Check sheet for the modelled part. Datum: model origin and axes. Units: mm. Face numbers are marked on the shaded views. A direction names the side the tool comes from. Round coordinates to 2 decimals unless told otherwise and drop trailing zeros. Write each loop counter-clockwise with the first axis right and the second up, starting at its lowest first coordinate (ties: lowest second). Pieces come first, ordered by that corner, then holes. Notation, with made-up numbers: (81.25, 35.25) - (131.25, 35.25) arc R24 ccw to (131.25, 61.25) - close; hole circle Ø9 at (-30.75, -13). An arc over 180 degrees is marked (long way). Answer as a JSON object with one key per item and string values. Group by question number.
Item 1: Sectioned sample at A-A on y = 0. Record the boundary of the cut face in (x, z), plus the area to 3 significant figures.
Item 2: Sectioned sample at D-D on y = -5.5. Record the boundary of the cut face in (x, z).
Item 3: Sectioned sample at C-C on x = 0. Record the boundary of the cut face in (y, z), plus the area to 3 significant figures.
Item 4: Sectioned sample at B-B on z = -35. Record the boundary of the cut face in (x, y), plus the area to 3 significant figures.
Item 5: Thickness scan on line 1 (Z direction, x = 4.5, y = -4.5); line 2 (X direction, y = 2.5, z = -33); line 3 (Y direction, x = 13.8, z = -35). Record the ranges inside material, lowest first.
Item 6: Gauge pin test, flat ends, axial feed: P1, Ø3.5, axis at x = 35.5, y = 2.5, coming from the +Z side; P2, Ø8, axis at y = 0, z = -35, coming from the +X side; P3, Ø6, axis at x = -35, z = 0, coming from the -Y side; P4, Ø1.5, axis at y = 5.5, z = 23, coming from the -X side. Record the tip position at first contact, or that the pin passes through.
Item 7: Release check for a two-part mould opening along X. For the marked faces 5, 6, 7 and 8 record: pulls with the +X half, pulls with the -X half, needs draft (parallel to the pull), parting line crosses it, or undercut.
Item 8: Set-up check for the marked faces 1, 2, 3 and 4: record each of +Z, -Z, +X, -X, +Y, -Y from which the full face is reachable in a straight line by a thin tool's end or side.
```python
from build123d import *

# Parameters (mm, degrees)
SCHIZZO1_R                    = 12
SCHIZZO1_R_2                  = 5
ESTRUSIONE_ESTRUSIONE1_DEPTH  = 7.5
TAGLIO_ESTRUSIONE1_DEPTH      = 73.284161474
TAGLIO_ESTRUSIONE1_DEPTH_BACK = 5
SCHIZZO3_R                    = 5
SCHIZZO4_R                    = 5
TAGLIO_ESTRUSIONE2_DEPTH      = 10
FORO_7_0_7_1_D                = 7
FORO_6_0_6_1_D                = 6


with BuildPart() as part:
    # Schizzo1 → Estrusione-Estrusione1 (new, symmetric)
    with BuildSketch(Plane(origin=(0, 0, 0), x_dir=(1, 0, 0), z_dir=(0, 1, 0))):
        with BuildLine():
            Line((-40, 30), (-16, 30))
            Line((-16, 30), (-16, 40))
            Line((-16, 40), (-10, 40))
            Line((-10, 40), (-10, 30))
            Line((-10, 30), (10, 30))
            Line((10, 30), (10, 40))
            Line((10, 40), (16, 40))
            Line((16, 40), (16, 30))
            Line((16, 30), (40, 30))
            ThreePointArc((40, 30), (0, -50), (-40, 30))
        make_face()
        with Locations(Location((0, 0, 0), (0, 0, 270))):
            Circle(SCHIZZO1_R, mode=Mode.SUBTRACT)
        with Locations(Location((0, -30, 0), (0, 0, 270))):
            Circle(SCHIZZO1_R_2, mode=Mode.SUBTRACT)
        with BuildLine():
            Line((29, 3), (41, 3))
            ThreePointArc((41, 3), (44, 0), (41, -3))
            Line((41, -3), (29, -3))
            ThreePointArc((29, -3), (26, 0), (29, 3))
        make_face(mode=Mode.SUBTRACT)
    extrude(amount=ESTRUSIONE_ESTRUSIONE1_DEPTH, both=True)

    # Schizzo3 → Taglio-Estrusione1 (cut, two sides: drawn at the far end of the back side and taken through both)
    # profile 1 of 2: a face of its own
    with BuildSketch(Plane(origin=(0, 7.5, 0), x_dir=(1, 0, 0), z_dir=(0, 1, 0)).offset(-TAGLIO_ESTRUSIONE1_DEPTH_BACK)):
        with BuildLine():
            Line((16.05, 0), (12, 0))
            ThreePointArc((12, 0), (0, -12), (-12, 0))
            Line((-12, 0), (-16.05, 0))
            Line((-16.05, 0), (-16.05, -47.353959708))
            ThreePointArc((-16.05, -47.353959708), (0, -50), (16.05, -47.353959708))
            Line((16.05, -47.353959708), (16.05, 0))
        make_face()
        with Locations(Location((0, -30, 0), (0, 0, 270))):
            Circle(SCHIZZO3_R, mode=Mode.SUBTRACT)
    # profile 2 of 2: a face of its own
    with BuildSketch(Plane(origin=(0, 7.5, 0), x_dir=(1, 0, 0), z_dir=(0, 1, 0)).offset(-TAGLIO_ESTRUSIONE1_DEPTH_BACK)):
        with BuildLine():
            ThreePointArc((-12, 0), (0, 12), (12, 0))
            Line((12, 0), (16.05, 0))
            ThreePointArc((16.05, 0), (0, 16.05), (-16.05, 0))
            Line((-16.05, 0), (-12, 0))
        make_face()
    extrude(amount=TAGLIO_ESTRUSIONE1_DEPTH + TAGLIO_ESTRUSIONE1_DEPTH_BACK, mode=Mode.SUBTRACT)

    # Schizzo4 → Taglio-Estrusione2 (cut)
    with BuildSketch(Plane(origin=(0, 7.5, 0), x_dir=(1, 0, 0), z_dir=(0, 1, 0))):
        with Locations(Location((-35, 0, 0), (0, 0, 270))):
            Circle(SCHIZZO4_R)
    extrude(amount=-TAGLIO_ESTRUSIONE2_DEPTH, mode=Mode.SUBTRACT)

    # Foro Ø7.0 (7)-1 (through all)
    with Locations(Plane(origin=(0, -2.5, 0), x_dir=(1, 0, 0), z_dir=(0, 1, 0))):
        with Locations((-35, 0)):
            Hole(FORO_7_0_7_1_D / 2)

    # Foro Ø6.0 (6)-1 (through all)
    with Locations(Plane.ZY.offset(16)):
        with Locations((-35, 0)):
            Hole(FORO_6_0_6_1_D / 2)


solid = part.part
```
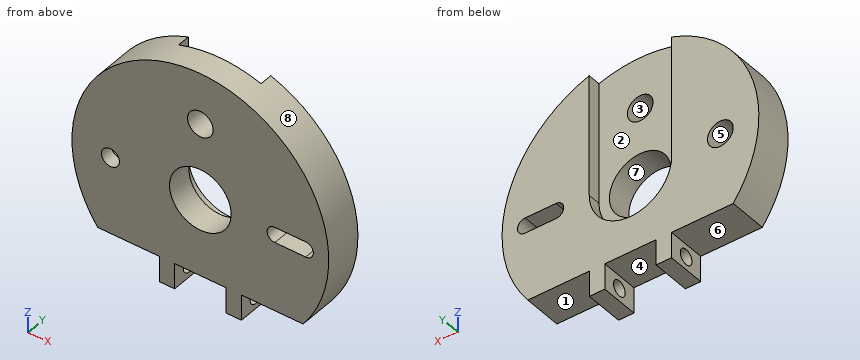
Completed:
{
 "1": {"outline": "(-40, -30) - (-16, -30) - (-16, -32) - (-10, -32) - (-10, -30) - (10, -30) - (10, -32) - (16, -32) - (16, -30) - (40, -30) arc R50 ccw (long way) to start; (-16, -40) - (-10, -40) - (-10, -38) - (-16, -38) - close; (10, -40) - (16, -40) - (16, -38) - (10, -38) - close; hole circle Ø10 at (-35, 0); hole circle Ø24 at (0, 0); hole circle Ø10 at (0, 30); hole (29, -3) - (41, -3) arc R3 ccw to (41, 3) - (29, 3) arc R3 ccw to start", "area": "6,070 mm²"},
 "2": {"outline": "(-40, -30) - (-16, -30) - (-16, -40) - (-10, -40) - (-10, -30) - (10, -30) - (10, -40) - (16, -40) - (16, -30) - (40, -30) arc R50 ccw (long way) to start; hole circle Ø7 at (-35, 0); hole circle Ø24 at (0, 0); hole circle Ø10 at (0, 30); hole (29, -3) - (41, -3) arc R3 ccw to (41, 3) - (29, 3) arc R3 ccw to start"},
 "3": {"outline": "(-7.5, -30) - (7.5, -30) - (7.5, -16.05) - (2.5, -16.05) - (2.5, -12) - (-7.5, -12) - close; (-7.5, 12) - (2.5, 12) - (2.5, 25) - (-7.5, 25) - close; (-7.5, 35) - (2.5, 35) - (2.5, 50) - (-7.5, 50) - close", "area": "530 mm²"},
 "4": {"outline": "(-16, -7.5) - (-10, -7.5) - (-10, -3) - (-16, -3) - close; (-16, 3) - (-10, 3) - (-10, 7.5) - (-16, 7.5) - close; (10, -7.5) - (16, -7.5) - (16, -3) - (10, -3) - close; (10, 3) - (16, 3) - (16, 7.5) - (10, 7.5) - close", "area": "108 mm²"},
 "5": {"line 1": "-30 to -11.12, 11.12 to 27.82, 32.18 to 49.8", "line 2": "-16 to -10, 10 to 16", "line 3": "-7.5 to -3, 3 to 7.5"},
 "6": {"P1": "z = 36.89", "P2": "x = 16", "P3": "through", "P4": "x = -44.78"},
 "7": {"face 5": "undercut", "face 6": "needs draft", "face 7": "undercut", "face 8": "parting line crosses it"},
 "8": {"face 1": "-Z, +X, +Y, -Y", "face 2": "+Z, +Y", "face 3": "+Y, -Y", "face 4": "-Z, +Y, -Y"}
}
